```python
from build123d import *

# Parameters (mm, degrees)
SKETCH1_W           = 11
SKETCH1_H           = 5.5
BOSS_EXTRUDE1_DEPTH = 1
BOSS_EXTRUDE2_DEPTH = 1
FILLET1_R           = 1


with BuildPart() as part:
    # Sketch1 → Boss-Extrude1 (new body)
    with BuildSketch(Plane(origin=(0, 0, 0), x_dir=(1, 0, 0), z_dir=(0, 1, 0))):
        Rectangle(SKETCH1_W, SKETCH1_H)
    extrude(amount=BOSS_EXTRUDE1_DEPTH)

    # Sketch2 → Boss-Extrude2 (add)
    with BuildSketch(Plane.XZ):
        with BuildLine():
            Line((6, 5), (-6, 5))
            ThreePointArc((-6, 5), (-7.414213562, 4.414213562), (-8, 3))
            Line((-8, 3), (-8, -3))
            ThreePointArc((-8, -3), (-7.414213562, -4.414213562), (-6, -5))
            Line((-6, -5), (6, -5))
            ThreePointArc((6, -5), (7.414213562, -4.414213562), (8, -3))
            Line((8, -3), (8, 3))
            ThreePointArc((8, 3), (7.414213562, 4.414213562), (6, 5))
        make_face()
    extrude(amount=BOSS_EXTRUDE2_DEPTH)

    # Fillet1
    fillet1_edges = [part.edges().sort_by_distance(p)[0] for p in [
        (5.5, 0.5, 2.75),
        (5.5, 0.5, -2.75),
        (-5.5, 0.5, -2.75),
        (-5.5, 0.5, 2.75),
    ]]
    fillet(fillet1_edges, radius=FILLET1_R)


solid = part.part
```
Read the model definition and answer for the solid it produces. Units are mm, in the model's axes. A direction names the side the tool comes from. Round coordinates to 2 decimals unless told otherwise and drop trailing zeros. Write each loop counter-clockwise with the first axis right and the second up, starting at its lowest first coordinate (ties: lowest second). Pieces come first, ordered by that corner, then holes. Notation, with made-up numbers: M -14.5,-33.75 L 39.5,-33.75 A26 ccw 39.5,2.25 Z; hole C 23.25,81.25 d10. An arc over 180 degrees is marked long. One line per item, written item: value.
Q1. Find section B-B on z = 0.75. Write down the section's boundary in (x, y), plus the area to 3 significant figures.
Data:
outline: M -8,-1 L 8,-1 L 8,0 L 5.5,0 L 5.5,1 L -5.5,1 L -5.5,0 L -8,0 Z
area: 27.0 mm2
Q2. Find section D-D on z = 3.5. Write down the section's boundary in (x, y), plus the area to 3 significant figures.
Data:
outline: M -7.94,-1 L 7.94,-1 L 7.94,0 L -7.94,0 Z
area: 15.9 mm2
Q3. Straight lines are drawn through the part: line 1 (Y direction, x = -2, z = 4.5); line 2 (X direction, y = 0.25, z = -1.5); line 3 (Z direction, x = -3, y = 0.35). For each, find the intervals that lie inside material, in ascending order. Write a range as [from, to].
Data:
line 1: [-1, 0]
line 2: [-5.5, 5.5]
line 3: [-2.75, 2.75]
Q4. Find section A-A on y = 0.25. Write down the section's boundary in (x, z).
Data:
outline: M -5.5,-1.75 A1 ccw -4.5,-2.75 L 4.5,-2.75 A1 ccw 5.5,-1.75 L 5.5,1.75 A1 ccw 4.5,2.75 L -4.5,2.75 A1 ccw -5.5,1.75 Z
Q5. Which of the six approach directions +Z, -Z, +X, -X, +Y, -Y give full straight-line access (tool end or side, diameter ignored) to faces 1 (the cylindrical face through (-5.215, 0.507, -2.449)), 2 (the flat face through (-0.1, 0.5, 2.75)), 3 (the flat face through (-5.5, 0.5, 0))?
Data:
face 1: -Z, -X, +Y
face 2: +Z, +X, -X, +Y
face 3: +Z, -Z, -X, +Y
Q6. Find section C-C on x = 5.75. Write down the section's boundary in (y, z).
Data:
outline: M -1,-5 L 0,-5 L 0,5 L -1,5 Z
Q7. Flat-ended cylindrical pins translate along their axes: pin 1 Ø0.8 at (x, y) = (0, 0.5) entering from -Z; pin 2 Ø0.5 at (y, z) = (0.5, 1) entering from +X; pin 3 Ø0.8 at (y, z) = (0.5, 1) entering from -X. Find the tip coordinate at first contact, or state that the pin passes through.
Data:
pin 1: z = -2.75
pin 2: x = 5.5
pin 3: x = -5.5
